The model under review builds one solid part; all positions refer to its coordinate system, in mm. Face numbers are marked on the shaded views. Round coordinates to 2 decimals unless told otherwise and drop trailing zeros. Order: outer loops, then holes, each group sorted by start corner. A loop starts at its lowest first (then second) coordinate and runs counter-clockwise, first axis right, second up.
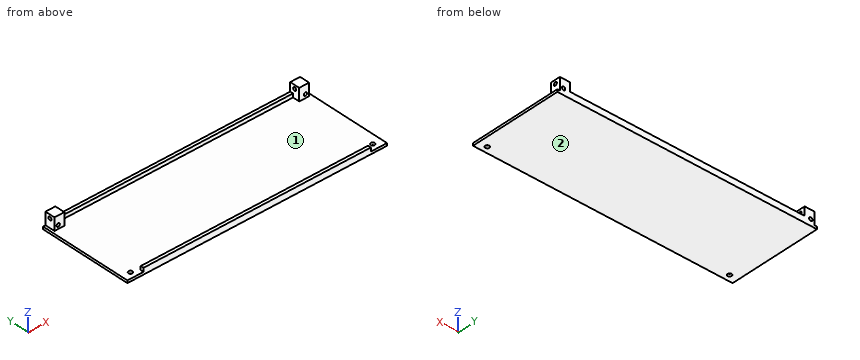
```python
from build123d import *

# Parameters (mm, degrees)
SKETCH1_W           = 210
SKETCH1_H           = 75
SKETCH1_R           = 1.65
BOSS_EXTRUDE1_DEPTH = 2
SKETCH2_W           = 8
SKETCH2_H           = 8
BOSS_EXTRUDE2_DEPTH = 10
SKETCH3_R           = 1.35
CUT_EXTRUDE1_DEPTH  = 10
SKETCH4_W           = 190
SKETCH4_H           = 2.5
BOSS_EXTRUDE3_DEPTH = 3
SKETCH5_W           = 184
SKETCH5_H           = 2.5
BOSS_EXTRUDE4_DEPTH = 3
SKETCH6_R           = 1.35
CUT_EXTRUDE2_DEPTH  = 209


with BuildPart() as part:
    # Sketch1 → Boss-Extrude1 (new body)
    with BuildSketch(Plane.XY):
        Rectangle(SKETCH1_W, SKETCH1_H)
        with Locations((-98, -32.5)):
            Circle(SKETCH1_R, mode=Mode.SUBTRACT)
        with Locations((98, -32.5)):
            Circle(SKETCH1_R, mode=Mode.SUBTRACT)
    extrude(amount=BOSS_EXTRUDE1_DEPTH)

    # Sketch2 → Boss-Extrude2 (add)
    with BuildSketch(Plane.XY.offset(2)):
        with Locations((-99, 33.5)):
            Rectangle(SKETCH2_W, SKETCH2_H)
        with Locations((99, 33.5)):
            Rectangle(SKETCH2_W, SKETCH2_H)
    extrude(amount=BOSS_EXTRUDE2_DEPTH)

    # Sketch3 → Cut-Extrude1 (cut)
    with BuildSketch(Plane(origin=(0, 37.5, 0), x_dir=(1, 0, 0), z_dir=(0, 1, 0))):
        with Locations((-100, -5)):
            Circle(SKETCH3_R)
        with Locations((100, -5)):
            Circle(SKETCH3_R)
    extrude(amount=-CUT_EXTRUDE1_DEPTH, mode=Mode.SUBTRACT)

    # Sketch4 → Boss-Extrude3 (add)
    with BuildSketch(Plane.XY.offset(2)):
        with Locations((0, 36.25)):
            Rectangle(SKETCH4_W, SKETCH4_H)
    extrude(amount=BOSS_EXTRUDE3_DEPTH)

    # Sketch5 → Boss-Extrude4 (add)
    with BuildSketch(Plane.XY.offset(2)):
        with Locations((0, -36.25)):
            Rectangle(SKETCH5_W, SKETCH5_H)
    extrude(amount=BOSS_EXTRUDE4_DEPTH)

    # Sketch6 → Cut-Extrude2 (cut, through all)
    with BuildSketch(Plane(origin=(103, 0, 0), x_dir=(0, 0, -1), z_dir=(1, 0, 0))):
        with Locations((-9, 33.5)):
            Circle(SKETCH6_R)
    extrude(amount=-CUT_EXTRUDE2_DEPTH, mode=Mode.SUBTRACT)


solid = part.part
```
(1) Insertion check: pin 1 (12 mm diameter, centred on x = -59, y = 13, fed in from +Z); pin 2 (2 mm diameter, centred on y = -36, z = 3.5, fed in from -X); pin 3 (4 mm diameter, centred on y = 33.5, z = 4.5, fed in from +X). Each pin has a flat end and moves straight along its axis. Give the tip position at first contact, or say it passes through.
Data:
pin 1: stops at z = 2
pin 2: stops at x = -92
pin 3: stops at x = 103
(2) Draft analysis for pull direction Y (two halves, no side actions). For the marked faces 1 and 2, state which applies: pulls with the +Y half, pulls with the -Y half, needs draft (parallel to the pull), parting line crosses it, or undercut.
Data:
face 1: undercut
face 2: needs draft
(3) To check wall thickness, follow probe 1 along X at (y, z) = (32.75, 5); probe 2 along Y at (x, z) = (-100.25, 9); probe 3 along Z at (x, y) = (100, 34). State the ranges of each line that lie inside material, in increasing order.
Data:
probe 1: x = -103 to -101.35, -98.65 to -95, 95 to 98.65, 101.35 to 103
probe 2: y = 29.5 to 32.15, 34.85 to 37.5
probe 3: z = 0 to 3.65, 6.35 to 7.75, 10.25 to 12
(4) Consider section B-B (y = 2). Write out the cut boundary in (x, z), and give its area (3 significant figures).
Data:
outline: (-105, 0) - (105, 0) - (105, 2) - (-105, 2) - close
area: 420 mm2
(5) Consider section A-A (x = 53.5). Write out the cut boundary in (y, z), and give its area (3 significant figures).
Data:
outline: (-37.5, 0) - (37.5, 0) - (37.5, 5) - (35, 5) - (35, 2) - (-35, 2) - (-35, 5) - (-37.5, 5) - close
area: 165 mm2
